```python
from build123d import *

# Parameters (mm, degrees)
F0_W      = 48.26
F0_H      = 48.26
F1_DEPTH  = 2.54
F2_W      = 12.7
F2_H      = 12.7
F3_DEPTH  = 1.27
F4_R      = 2.8715074031
F5_DEPTH  = 50.8
F6_R      = 0.3093193385
F6_R_2    = 0.3272888375
F6_R_3    = 0.3568571673
F6_R_4    = 0.3525339216
F7_DEPTH  = 0.762
F8_R      = 0.254
F12_W     = 0.0615678008
F12_H     = 0.0203329791
F12_W_2   = 0.0220249466
F12_H_2   = 0.0622902502
F11_W     = 0.0480206565
F11_H     = 0.0132349783
F11_W_2   = 0.0138029049
F11_H_2   = 0.0482696602
F10_W     = 0.0884033393
F10_H     = 0.017505979
F10_W_2   = 0.0194820769
F10_H_2   = 0.0892982516
F9_W      = 0.0940955169
F9_H      = 0.0154326007
F9_W_2    = 0.0169436104
F9_H_2    = 0.0947913842
F13_DEPTH = 0.508
F15_DEPTH = 1.41478
F16_R     = 0.9021855569
F17_DEPTH = 19.05
F19_DEPTH = 1.016
F20_R     = 0.8982139902
F21_DEPTH = 19.05
F23_DEPTH = 1.27
F24_R     = 0.9025250594
F25_DEPTH = 19.05
F27_DEPTH = 1.19634
F28_R     = 0.8978475469
F29_DEPTH = 19.05


with BuildPart() as f1:
    # F0 (on Top) → F1 (new body)
    with BuildSketch(Plane.XY):
        Rectangle(F0_W, F0_H)
    extrude(amount=F1_DEPTH)

    # F2 (on face) → F3 (join)
    with BuildSketch(Plane(origin=(0, 0, 0), x_dir=(1, 0, 0), z_dir=(0, 0, -1))):
        Rectangle(F2_W, F2_H)
    extrude(amount=F3_DEPTH)

    # F4 (on face) → F5 (join)
    with BuildSketch(Plane(origin=(0, 0, -1.27), x_dir=(1, 0, 0), z_dir=(0, 0, -1))):
        with Locations((0.0108288368, 0.0445277688)):
            Circle(F4_R)
    extrude(amount=F5_DEPTH)

    # F6 (on face) → F7 (join)
    with BuildSketch(Plane(origin=(0, 0, -1.27), x_dir=(1, 0, 0), z_dir=(0, 0, -1))):
        with Locations((-5.7706111111, 5.6873215362)):
            Circle(F6_R)
        with Locations((-5.7180044241, -5.6720911525)):
            Circle(F6_R_2)
        with Locations((5.6732143275, -5.739856977)):
            Circle(F6_R_3)
        with Locations((5.6450250559, 5.5452911183)):
            Circle(F6_R_4)
    extrude(amount=F7_DEPTH)

    # F8
    f8_edges = [f1.edges().sort_by_distance(p)[0] for p in [
        (-6.07993, -5.687322, -2.032),
        (5.316357, 5.739857, -2.032),
        (-6.045293, 5.672091, -2.032),
        (5.292491, -5.545291, -2.032),
    ]]
    fillet(f8_edges, radius=F8_R)

    # F12 (on face) + F11 (on face) + F10 (on face) + F9 (on face) → F13 (cut)
    with BuildSketch(Plane(origin=(0, 0, -2.032), x_dir=(1, 0, 0), z_dir=(0, 0, -1))):
        with Locations((-5.6762080504, -5.6720911525)):
            Rectangle(F12_W, F12_H)
        with Locations((-5.7180044241, -5.7134027672)):
            Rectangle(F12_W_2, F12_H_2)
        with Locations((-5.7180044241, -5.6720911525)):
            Rectangle(F12_W_2, F12_H)
        with Locations((-5.7598007978, -5.6720911525)):
            Rectangle(F12_W, F12_H)
        with Locations((-5.7180044241, -5.6307795379)):
            Rectangle(F12_W_2, F12_H_2)
    with BuildSketch(Plane(origin=(0, 0, -2.032), x_dir=(1, 0, 0), z_dir=(0, 0, -1))):
        with Locations((-5.8015228918, 5.6873215362)):
            Rectangle(F11_W, F11_H)
        with Locations((-5.7396993304, 5.6873215362)):
            Rectangle(F11_W, F11_H)
        with Locations((-5.7706111111, 5.6873215362)):
            Rectangle(F11_W_2, F11_H)
        with Locations((-5.7706111111, 5.656569217)):
            Rectangle(F11_W_2, F11_H_2)
        with Locations((-5.7706111111, 5.7180738555)):
            Rectangle(F11_W_2, F11_H_2)
    with BuildSketch(Plane(origin=(0, 0, -2.032), x_dir=(1, 0, 0), z_dir=(0, 0, -1))):
        with Locations((5.6989677639, 5.5452911183)):
            Rectangle(F10_W, F10_H)
        with Locations((5.6450250559, 5.491889003)):
            Rectangle(F10_W_2, F10_H_2)
        with Locations((5.6450250559, 5.5452911183)):
            Rectangle(F10_W_2, F10_H)
        with Locations((5.5910823478, 5.5452911183)):
            Rectangle(F10_W, F10_H)
        with Locations((5.6450250559, 5.5986932336)):
            Rectangle(F10_W_2, F10_H_2)
    with BuildSketch(Plane(origin=(0, 0, -2.032), x_dir=(1, 0, 0), z_dir=(0, 0, -1))):
        with Locations((5.7287338912, -5.739856977)):
            Rectangle(F9_W, F9_H)
        with Locations((5.6732143275, -5.7949689694)):
            Rectangle(F9_W_2, F9_H_2)
        with Locations((5.6732143275, -5.739856977)):
            Rectangle(F9_W_2, F9_H)
        with Locations((5.6176947639, -5.739856977)):
            Rectangle(F9_W, F9_H)
        with Locations((5.6732143275, -5.6847449846)):
            Rectangle(F9_W_2, F9_H_2)
    extrude(amount=-F13_DEPTH, mode=Mode.SUBTRACT)

    # F14 (on face) → F15 (cut)
    with BuildSketch(Plane(origin=(0, 0, -52.07), x_dir=(1, 0, 0), z_dir=(0, 0, -1))):
        Polygon((0, 3.2037144993), (-0.6241711632, 2.8449437675), (0.6458288368, 2.8449437675), align=None)
    extrude(amount=-F15_DEPTH, mode=Mode.SUBTRACT)

    # F16 (on face) → F17 (join)
    with BuildSketch(Plane.XZ.offset(2.8449437675)):
        with Locations((0, -51.1687509716)):
            Circle(F16_R)
    extrude(amount=F17_DEPTH)

    # F18 (on face) → F19 (cut)
    with BuildSketch(Plane(origin=(0, 0, -52.07), x_dir=(1, 0, 0), z_dir=(0, 0, -1))):
        Polygon((3.0578877777, 0), (2.8145416692, 0.6648092527), (2.8078707354, -0.6051732269), align=None)
    extrude(amount=-F19_DEPTH, mode=Mode.SUBTRACT)

    # F20 (on face) → F21 (join)
    with BuildSketch(Plane(origin=(2.8109720156, 0.0147654072, 0), x_dir=(-0.0052527038, 0.9999862045, 0), z_dir=(0.9999862045, 0.0052527038, 0))):
        with Locations((0, -51.2162931263)):
            Circle(F20_R)
    extrude(amount=F21_DEPTH)

    # F22 (on face) → F23 (cut)
    with BuildSketch(Plane(origin=(0, 0, -52.07), x_dir=(1, 0, 0), z_dir=(0, 0, -1))):
        Polygon((0.6786663537, -2.7482392851), (-0.6570086801, -2.7482392851), (0, -2.9700854793), align=None)
    extrude(amount=-F23_DEPTH, mode=Mode.SUBTRACT)

    # F24 (on face) → F25 (join)
    with BuildSketch(Plane(origin=(0, 2.7482392851, 0), x_dir=(-1, 0, 0), z_dir=(0, 1, 0))):
        with Locations((0, -51.1333122849)):
            Circle(F24_R)
    extrude(amount=F25_DEPTH)

    # F26 (on face) → F27 (cut)
    with BuildSketch(Plane(origin=(0, 0, -52.07), x_dir=(1, 0, 0), z_dir=(0, 0, -1))):
        Polygon((-2.8074634724, -0.5057296489), (-2.8154312504, 0), (-2.8233990284, 0.5057296489), (-2.9956893995, 0), align=None)
    extrude(amount=-F27_DEPTH, mode=Mode.SUBTRACT)

    # F28 (on face) → F29 (join)
    with BuildSketch(Plane(origin=(-2.8147325761, 0.0443461527, 0), x_dir=(-0.0157530595, -0.9998759129, 0), z_dir=(-0.9998759129, 0.0157530595, 0))):
        with Locations((0, -51.189865917)):
            Circle(F28_R)
    extrude(amount=F29_DEPTH)


solid = f1.part
```
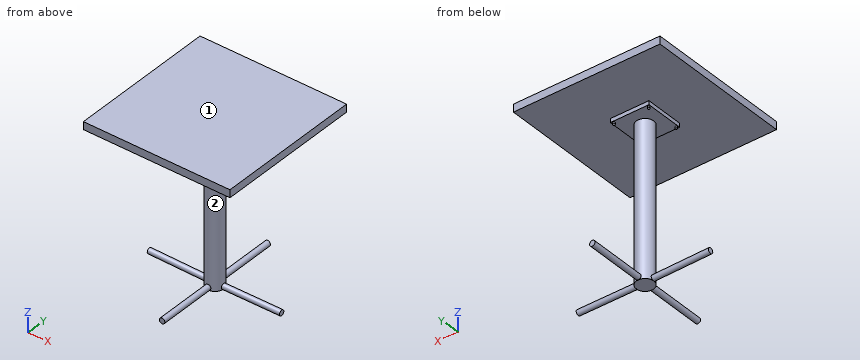
Model file for the job. Use its own axes, mm. Face numbers are marked on the shaded views. Give positions to 0.01 mm unless a question says otherwise; leave off trailing zeros. Loops run counter-clockwise (first coordinate to the right, second up) from the corner with the lowest first, then second, coordinate; pieces in that order, holes last. Notation, with made-up numbers: (25, 45) -> (54, 45) arc R15 cw to (54, 60) -> close; hole circle Ø10 at (37, 46.5). An arc over 180 degrees is marked (long way). Write each question's results on one line, items separated by ' | '.
(1) Probe line 1 along Z through (x, y) = (21, 2); line 2 along Z through (x, y) = (2, 5.5); line 3 along Y through (x, z) = (-2, -7.5). List the from-to ranges inside material, lowest first.
Geometry results:
line 1: z = 0 to 2.54 | line 2: z = -1.27 to 2.54 | line 3: y = -2.09 to 2.01
(2) Flat gauge pins, fed straight in: pin 1 Ø1 at (x, y) = (17, 8.5) entering from -Z; pin 2 Ø10 at (y, z) = (4, -27) entering from -X; pin 3 Ø3 at (x, y) = (0.5, -0.5) entering from -Z. Where does each tip first touch, or does it go through?
Geometry results:
pin 1: stops at z = 0 | pin 2: stops at x = -2.86 | pin 3: stops at z = -52.07
(3) Cut at D-D on y = 11. List the corners of the cut face in (x, z).
Geometry results:
outline: (-24.13, 0) -> (24.13, 0) -> (24.13, 2.54) -> (-24.13, 2.54) -> close; circle Ø1.81 at (0, -51.13)
(4) Pull direction Z, two halves, no side cores. Call the marked faces 1 and 2: released by +Z, released by -Z, zero draft, split by the parting line, or undercut.
Geometry results:
face 1: released by +Z | face 2: undercut
(5) Cut at A-A on y = -4. List the corners of the cut face in (x, z).
Geometry results:
outline: (-24.13, 0) -> (-6.35, 0) -> (-6.35, -1.27) -> (6.35, -1.27) -> (6.35, 0) -> (24.13, 0) -> (24.13, 2.54) -> (-24.13, 2.54) -> close; circle Ø1.8 at (0, -51.17)
(6) Cut at B-B on y = -17. List the corners of the cut face in (x, z), and give its area (3 significant figures).
Geometry results:
outline: (-24.13, 0) -> (24.13, 0) -> (24.13, 2.54) -> (-24.13, 2.54) -> close; circle Ø1.8 at (0, -51.17) | area: 125 mm²
(7) Cut at C-C on z = -10. List the corners of the cut face in (x, y), and give its area (3 significant figures).
Geometry results:
outline: circle Ø5.74 at (0.01, -0.04) | area: 25.9 mm²
